Design review of the part built by this model. Coordinates are the model's own, in mm. A direction names the side the tool comes from. Coordinates: 2 decimals unless noted, no trailing zeros. Loops run counter-clockwise (first coordinate to the right, second up) from the corner with the lowest first, then second, coordinate; pieces in that order, holes last. Notation, with made-up numbers: M 86.25,15 L 141.25,15 A28 cw 141.25,45 Z; hole C 77.25,-4 d9. An arc over 180 degrees is marked long. Answer as a JSON object with one key per item and string values. Group by question number.
1. To check wall thickness, follow probe 1 along Y at (x, z) = (-25.4, 6) (3 decimals); probe 2 along Y at (x, z) = (-5, 3) (3 decimals); probe 3 along Y at (x, z) = (-2.5, 25) (3 decimals). State the ranges of each line that lie inside material, in increasing order.
2. Draft analysis for pull direction Y (two halves, no side actions). For faces 1 (the flat face through (-20, -41.275, 22)), 2 (the flat face through (-10, -101.6, 22)), 3 (the flat face through (-50.8, -50, 22)), state which applies: +Y half, -Y half, draft (parallel to the pull), parting line (faces both ways), or undercut.
3. Consider section A-A (y = -69.85). State the section outline as (x, z) points (3 decimals).
4. Consider section C-C (y = -31.75). State the section outline as (x, z) points, then the cut area to 3 significant figures.
5. Insertion check: pin 1 (4 mm diameter, centred on x = -12.7, z = 22.225, fed in from +Y) (3 decimals); pin 2 (6 mm diameter, centred on x = -25.4, y = -69.85, fed in from -Z); pin 3 (15 mm diameter, centred on y = -33.5, z = 15.5, fed in from +X). Each pin has a flat end and moves straight along its axis. Give the tip position at first contact, or say it passes through.
6. Consider section D-D (z = 39.5). State the section outline as (x, y) points (3 decimals).
7. Machinability: for faces 4 (the flat face through (-26, -50, 0)), 5 (the flat face through (-19, -22.225, 22)), 6 (the cylindrical face through (-10.644, -11.268, 19.544)), which of the approach directions +Z, -Z, +X, -X, +Y, -Y give a long, thin tool a straight path to every point of the face, cutting with its end or side? Answer none if there is none.
8. Consider section B-B (x = -25.4). State the section outline as (y, z) points (3 decimals), then the cut area to 3 significant figures.
Autodesk Inventor part; units mm, degrees
ref_plane "YZ Plane" through (0, 0, 0) normal (1, 0, 0) x (0, 1, 0)
ref_plane "XZ Plane" through (0, 0, 0) normal (0, 1, 0) x (-1, 0, 0)
ref_plane "XY Plane" through (0, 0, 0) normal (0, 0, 1) x (1, 0, 0)
sketch "Sketch1" plane through (0, 0, 0) normal (0, 0, 1) x (1, 0, 0)
  line L0 (0, 0) -> (-50.8, 0)
  line L1 (-50.8, 0) -> (-50.8, -101.6)
  line L2 (-50.8, -101.6) -> (0, -101.6)
  line L3 (0, -22.225) -> (-38.1, -22.225)
  line L4 (-38.1, -22.225) -> (-38.1, -41.275)
  line L5 (-38.1, -41.275) -> (0, -41.275)
  line L6 (0, -101.6) -> (0, -41.275)
  line L7 (0, -22.225) -> (0, 0)
  dimension "d0" = 101.6
  dimension "d1" = 50.8
  dimension "d4" = 22.225
  dimension "d5" = 38.1
  dimension "d6" = 19.05
extrude "Extrusion1" add sketch "Sketch1" along normal blind 44.45
sketch "Sketch2" plane through (0, -22.225, 0) normal (1, 0, 0) x (0, 0, -1)
  line L0 (-44.45, 0) -> (-44.45, 22.225)
  line L1 (0, 22.225) -> (0, -79.375)
  line L2 (-44.45, 22.225) -> (0, 22.225)
  line L3 (0, 22.225) -> (0, -79.375)
  line L4 (0, -79.375) -> (-44.45, -79.375)
  line L5 (-44.45, -79.375) -> (-44.45, 22.225)
extrude "Extrusion2" cut sketch "Sketch2" against normal blind 0.381
sketch "Sketch3" plane through (-50.8, 0, 44.45) normal (0, 1, 0) x (1, 0, 0)
  line L0 (0, 44.45) -> (0, 0)
  line L1 (50.419, 44.45) -> (0, 44.45)
  point P0 (50.8, 44.45)
  point P1 (38.1, 22.225)
  dimension "d9" = 38.1
  dimension "d10" = 22.225
hole "Hole1" at (-12.7, 0, 22.225) direction (0, -1, 0) diameter 6.7564 end up to surface
sketch "Sketch4" plane through (-50.8, -101.6, 0) normal (-1, 0, 0) x (0, 0, 1)
  line L0 (0, 101.6) -> (0, 0)
  line L1 (0, 101.6) -> (44.45, 101.6)
  point P0 (22.225, 69.85)
  dimension "d18" = 22.225
  dimension "d19" = 31.75
hole "Hole2" at (-50.8, -31.75, 22.225) direction (1, 0, 0) diameter 6.7564 end through all
sketch "Sketch5" plane through (-50.8, -101.6, 0) normal (-1, 0, 0) x (0, 0, 1)
  line L0 (0, 101.6) -> (0, 0)
  line L1 (0, 101.6) -> (44.45, 101.6)
  point P0 (22.225, 31.75)
  dimension "d27" = 22.225
  dimension "d28" = 69.85
hole "Hole3" at (-50.8, -69.85, 22.225) direction (1, 0, 0) diameter 25.4 end through all
sketch "Sketch6" plane through (0, 0, 44.45) normal (0, 0, 1) x (1, 0, 0)
  line L0 (-0.381, 0) -> (-50.8, 0)
  line L1 (-50.8, 0) -> (-50.8, -101.6)
  point P0 (0, 0)
  point P1 (-25.4, -69.85)
  dimension "d36" = 69.85
  dimension "d37" = 25.4
hole "Hole4" at (-25.4, -69.85, 44.45) direction (0, 0, -1) diameter 6.7564 end through all
sketch "Sketch7" plane through (0, 0, 44.45) normal (0, 0, 1) x (1, 0, 0)
  circle A0 centre (-25.4, -101.6) radius 6.35
  line L0 (-0.381, 0) -> (-50.8, 0)
  line L1 (-50.8, 0) -> (-50.8, -101.6)
  point P0 (0, 0)
  dimension "d45" = 101.6
  dimension "d46" = 25.4
  dimension "d47" = 12.7
extrude "Extrusion3" cut sketch "Sketch7" against normal through all
properties part number "AsBuilt Over Support For Arm"
Findings below:
{
 "1": {"probe 1": "y = -95.25 to -73.228, -66.472 to -41.275, -22.225 to 0", "probe 2": "y = -101.6 to -41.275, -22.225 to 0", "probe 3": "y = -101.6 to -82.243, -57.457 to -41.275, -22.225 to 0"},
 "2": {"face 1": "undercut", "face 2": "-Y half", "face 3": "draft"},
 "3": {"outline": "M -50.8,0 L -28.778,0 L -28.778,9.525 L -50.8,9.525 Z; M -50.8,34.925 L -28.778,34.925 L -28.778,44.45 L -50.8,44.45 Z; M -22.022,0 L -0.381,0 L -0.381,9.525 L -22.022,9.525 Z; M -22.022,34.925 L -0.381,34.925 L -0.381,44.45 L -22.022,44.45 Z"},
 "4": {"outline": "M -50.8,0 L -38.1,0 L -38.1,18.85 L -50.8,18.85 Z; M -50.8,25.6 L -38.1,25.6 L -38.1,44.45 L -50.8,44.45 Z", "area": "479 mm^2"},
 "5": {"pin 1": "stops at y = -41.275", "pin 2": "passes through", "pin 3": "stops at x = -38.1"},
 "6": {"outline": "M -50.8,-101.6 L -31.75,-101.6 A6.35 cw -19.05,-101.6 L -0.381,-101.6 L -0.381,-41.275 L -38.1,-41.275 L -38.1,-22.225 L -0.381,-22.225 L -0.381,0 L -50.8,0 Z; hole C -25.4,-69.85 d6.756"},
 "7": {"face 4": "-Z, +X, -X, +Y, -Y", "face 5": "+Z, -Z, +X", "face 6": "+Y"},
 "8": {"outline": "M -95.25,0 L -73.228,0 L -73.228,9.983 A12.7 cw -73.228,34.467 L -73.228,44.45 L -95.25,44.45 Z; M -66.472,0 L -41.275,0 L -41.275,44.45 L -66.472,44.45 L -66.472,34.467 A12.7 cw -66.472,9.983 Z; M -22.225,0 L 0,0 L 0,44.45 L -22.225,44.45 Z", "area": "2,750 mm^2"}
}
